```python
from build123d import *

# Parameters (mm, degrees)
SKETCH1_W           = 192.0875
SKETCH1_H           = 95.9358
BOSS_EXTRUDE1_DEPTH = 13.1826
SKETCH2_W           = 166.1795
SKETCH2_H           = 70.0278
CUT_EXTRUDE1_DEPTH  = 7.874
SKETCH3_R           = 1.27
CUT_EXTRUDE2_DEPTH  = 7.874
SKETCH4_W           = 15.7988
SKETCH4_H           = 8.2804
BOSS_EXTRUDE2_DEPTH = 9.8298
SKETCH5_W           = 8.89
SKETCH5_H           = 27.94
BOSS_EXTRUDE3_DEPTH = 7.874
SKETCH6_R           = 1.0668
BOSS_EXTRUDE4_DEPTH = 3.683
FILLET1_R           = 5.08
FILLET2_R           = 0.635


with BuildPart() as part:
    # Sketch1 → Boss-Extrude1 (new body)
    with BuildSketch(Plane(origin=(0, 0, 0), x_dir=(1, 0, 0), z_dir=(0, 1, 0))):
        with Locations((96.04375, 47.9679)):
            Rectangle(SKETCH1_W, SKETCH1_H)
    extrude(amount=BOSS_EXTRUDE1_DEPTH)

    # Sketch2 → Cut-Extrude1 (cut)
    with BuildSketch(Plane.XZ):
        with Locations((96.04375, -47.9679)):
            Rectangle(SKETCH2_W, SKETCH2_H)
    extrude(amount=-CUT_EXTRUDE1_DEPTH, mode=Mode.SUBTRACT)

    # Sketch3 → Cut-Extrude2 (cut)
    with BuildSketch(Plane.XZ):
        with Locations((12.7, -85.7758)):
            Circle(SKETCH3_R)
        with Locations((12.7, -10.16)):
            Circle(SKETCH3_R)
        with Locations((179.3875, -85.7758)):
            Circle(SKETCH3_R)
        with Locations((179.3875, -10.16)):
            Circle(SKETCH3_R)
    extrude(amount=-CUT_EXTRUDE2_DEPTH, mode=Mode.SUBTRACT)

    # Sketch4 → Boss-Extrude2 (add)
    with BuildSketch(Plane(origin=(0, 7.874, 0), x_dir=(-1, 0, 0), z_dir=(0, -1, 0))):
        with Locations((-74.1934, 49.8094)):
            Rectangle(SKETCH4_W, SKETCH4_H)
    extrude(amount=BOSS_EXTRUDE2_DEPTH)

    # Sketch5 → Boss-Extrude3 (add)
    with BuildSketch(Plane(origin=(0, 7.874, 0), x_dir=(-1, 0, 0), z_dir=(0, -1, 0))):
        with Locations((-21.2598, 48.387)):
            Rectangle(SKETCH5_W, SKETCH5_H)
        with Locations((-170.8277, 48.387)):
            Rectangle(SKETCH5_W, SKETCH5_H)
    extrude(amount=BOSS_EXTRUDE3_DEPTH)

    # Sketch6 → Boss-Extrude4 (add)
    with BuildSketch(Plane(origin=(0, 0, 0), x_dir=(-1, 0, 0), z_dir=(0, -1, 0))):
        with Locations((-8.2804, 17.8562)):
            Circle(SKETCH6_R)
        with Locations((-183.8071, 78.0796)):
            Circle(SKETCH6_R)
    extrude(amount=BOSS_EXTRUDE4_DEPTH)

    # Fillet1
    fillet1_edges = [part.edges().sort_by_distance(p)[0] for p in [
        (12.954, 3.937, -82.9818),
        (12.954, 3.937, -12.954),
        (179.1335, 3.937, -12.954),
        (179.1335, 3.937, -82.9818),
    ]]
    fillet(fillet1_edges, radius=FILLET1_R)

    # Fillet2
    fillet2_edges = [part.edges().sort_by_distance(p)[0] for p in [
        (9.3472, -3.683, -17.8562),
        (184.8739, -3.683, -78.0796),
    ]]
    fillet(fillet2_edges, radius=FILLET2_R)


solid = part.part
```
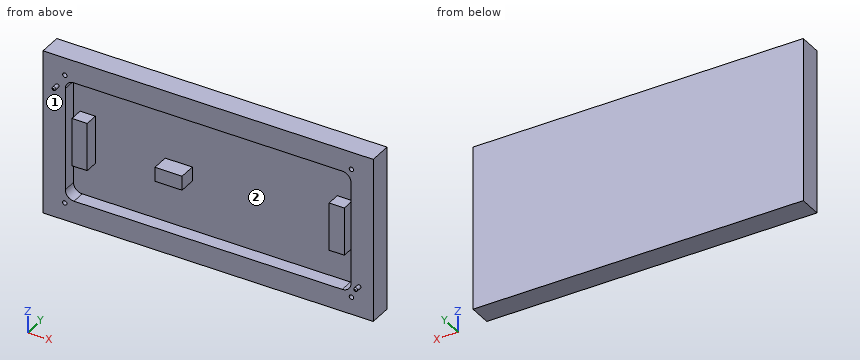
The listing builds one solid part. Answer for the finished solid, in the listing's coordinates (mm). Face numbers are marked on the shaded views. Coordinates: 2 decimals unless noted, no trailing zeros. Loops run counter-clockwise (first coordinate to the right, second up) from the corner with the lowest first, then second, coordinate; pieces in that order, holes last. Notation, with made-up numbers: (50.25, -27) - (81.25, -27) arc R29 cw to (81.25, 8) - close; hole circle Ø9 at (-34.5, 7). An arc over 180 degrees is marked (long way). Use a Markdown table: item, result. Add a question column.
1) Given pin 1 (6 mm diameter, centred on x = 76, z = -79.5, fed in from -Y); pin 2 (2.5 mm diameter, centred on x = 169.5, z = -55, fed in from -Y), each flat-ended and moving along its own axis, determine where each tip first touches the part or whether it passes through.
2) Find the intervals of material crossed by line 1 (X direction, y = 7.75, z = -57.5); line 2 (Z direction, x = 12.7, y = 5); line 3 (X direction, y = 6.75, z = -28), in increasing order.
3) The part is cut by section B-B, the plane x = 72.5. Give the vertices of the cut face in (y, z).
4) The mould has two halves that part along Z. Classify the marked faces 1 and 2: released by +Z, released by -Z, zero draft, split by the parting line, or undercut.
5) The part is cut by section A-A, the plane z = -58.5. Give the vertices of the cut face in (x, y), and give its area (3 significant figures).
Here are the results:
| question | item | result |
|---|---|---|
| 1 | pin 1 | stops at y = 7.87 |
| 1 | pin 2 | stops at y = 0 |
| 2 | line 1 | x = 0 to 12.95, 16.81 to 25.7, 166.38 to 175.27, 179.13 to 192.09 |
| 2 | line 2 | z = -95.94 to -87.05, -84.51 to -11.43, -8.89 to 0 |
| 2 | line 3 | x = 0 to 12.95, 179.13 to 192.09 |
| 3 | outline | (-1.96, -53.95) - (7.87, -53.95) - (7.87, -82.98) - (0, -82.98) - (0, -95.94) - (13.18, -95.94) - (13.18, 0) - (0, 0) - (0, -12.95) - (7.87, -12.95) - (7.87, -45.67) - (-1.96, -45.67) - close |
| 4 | face 1 | zero draft |
| 4 | face 2 | undercut |
| 5 | outline | (0, 0) - (12.95, 0) - (12.95, 7.87) - (16.81, 7.87) - (16.81, 0) - (25.7, 0) - (25.7, 7.87) - (166.38, 7.87) - (166.38, 0) - (175.27, 0) - (175.27, 7.87) - (179.13, 7.87) - (179.13, 0) - (192.09, 0) - (192.09, 13.18) - (0, 13.18) - close |
| 5 | area | 1,360 mm^2 |
